Design review of the part built by this model. Coordinates are the model's own, in mm. A direction names the side the tool comes from. Give positions to 0.01 mm unless a question says otherwise; leave off trailing zeros. Loops run counter-clockwise (first coordinate to the right, second up) from the corner with the lowest first, then second, coordinate; pieces in that order, holes last. Notation, with made-up numbers: (83, 69.25) - (112, 69.25) arc R16 cw to (112, 81.25) - close; hole circle Ø10 at (34, -2.75). An arc over 180 degrees is marked (long way). One line per item, written item: value. Start each with the question number.
```python
from build123d import *

# Parameters (mm, degrees)
SKETCH_1_W      = 22
SKETCH_1_H      = 14
SKETCH_1_R      = 1.5
SKETCH_1_W_2    = 11
SKETCH_1_H_2    = 6
EXTRUDE_1_DEPTH = 2.5
FILLET_1_R      = 2


with BuildPart() as part:
    # 草图1 → 凸台-拉伸1 (new body)
    with BuildSketch(Plane.XY):
        Rectangle(SKETCH_1_W, SKETCH_1_H)
        with Locations((8, 4)):
            Circle(SKETCH_1_R, mode=Mode.SUBTRACT)
        with Locations((8, -4)):
            Circle(SKETCH_1_R, mode=Mode.SUBTRACT)
        with Locations((-8, -4)):
            Circle(SKETCH_1_R, mode=Mode.SUBTRACT)
        with Locations((-8, 4)):
            Circle(SKETCH_1_R, mode=Mode.SUBTRACT)
        Rectangle(SKETCH_1_W_2, SKETCH_1_H_2, mode=Mode.SUBTRACT)
    extrude(amount=EXTRUDE_1_DEPTH)

    # 圆角1
    fillet_1_edges = [part.edges().sort_by_distance(p)[0] for p in [
        (5.5, -3, 1.25),
        (5.5, 3, 1.25),
        (-5.5, 3, 1.25),
        (-5.5, -3, 1.25),
        (11, -7, 1.25),
        (-11, -7, 1.25),
        (-11, 7, 1.25),
        (11, 7, 1.25),
    ]]
    fillet(fillet_1_edges, radius=FILLET_1_R)


solid = part.part
```
(1) Take a section at C-C on y = 0. State the section outline as (x, z) points.
(2) For pin 1 Ø1.8 at (x, y) = (8, -4) entering from +Z; pin 2 Ø1.5 at (x, y) = (5.5, -4.5) entering from -Z, all flat-tipped, find the tip position at first contact; note any pin that passes through.
(3) Take a section at B-B on x = -8. State the section outline as (y, z) points, and give its area (3 significant figures).
(4) Take a section at A-A on y = 4. State the section outline as (x, z) points.
(5) Draft analysis for pull direction X (two halves, no side actions). For faces 1 (the flat face through (-0.2, 3.2, 2.5)), 2 (the flat face through (11, 0, 1)), 3 (the cylindrical face through (-9.5, 4.07, 1.23)), 4 (the cylindrical face through (4.93, 2.4, 1.27)), state which applies: pulls with the +X half, pulls with the -X half, needs draft (parallel to the pull), parting line crosses it, or undercut.
(6) Machinability: for faces 5 (the flat face through (0, 7, 1)), 6 (the cylindrical face through (4.9, -2.43, 1.27)), which of the approach directions +Z, -Z, +X, -X, +Y, -Y give a long, thin tool a straight path to every point of the face, cutting with its end or side? Answer none if there is none.
(7) Take a section at D-D on z = 1.7. State the section outline as (x, y) points.
(8) To check wall thickness, follow L1, parallel to Y at x = -8, z = 1; L2, parallel to Y at x = 3, z = 0.85; L3, parallel to Y at x = -6.75, z = 1.1. State the ranges of each line that lie inside material, in increasing order. Write a range as from..to.
Here are the results:
1. outline: (-11, 0) - (-5.5, 0) - (-5.5, 2.5) - (-11, 2.5) - close; (5.5, 0) - (11, 0) - (11, 2.5) - (5.5, 2.5) - close
2. pin 1: through
2. pin 2: z = 0
3. outline: (-7, 0) - (-5.5, 0) - (-5.5, 2.5) - (-7, 2.5) - close; (-2.5, 0) - (2.5, 0) - (2.5, 2.5) - (-2.5, 2.5) - close; (5.5, 0) - (7, 0) - (7, 2.5) - (5.5, 2.5) - close
3. area: 20.0 mm²
4. outline: (-11, 0) - (-9.5, 0) - (-9.5, 2.5) - (-11, 2.5) - close; (-6.5, 0) - (6.5, 0) - (6.5, 2.5) - (-6.5, 2.5) - close; (9.5, 0) - (11, 0) - (11, 2.5) - (9.5, 2.5) - close
5. face 1: needs draft
5. face 2: pulls with the +X half
5. face 3: undercut
5. face 4: undercut
6. face 5: +Z, -Z, +X, -X, +Y
6. face 6: +Z, -Z
7. outline: (-11, -5) arc R2 ccw to (-9, -7) - (9, -7) arc R2 ccw to (11, -5) - (11, 5) arc R2 ccw to (9, 7) - (-9, 7) arc R2 ccw to (-11, 5) - close; hole circle Ø3 at (-8, -4); hole circle Ø3 at (-8, 4); hole (-5.5, -1) arc R2 ccw to (-3.5, -3) - (3.5, -3) arc R2 ccw to (5.5, -1) - (5.5, 1) arc R2 ccw to (3.5, 3) - (-3.5, 3) arc R2 ccw to (-5.5, 1) - close; hole circle Ø3 at (8, -4); hole circle Ø3 at (8, 4)
8. L1: -7..-5.5, -2.5..2.5, 5.5..7
8. L2: -7..-3, 3..7
8. L3: -7..-4.83, -3.17..3.17, 4.83..7
